from build123d import *

# Parameters (mm, degrees)
F1_DEPTH = 2.54


with BuildPart() as f1:
    # F0 (on Front) → F1 (new body, symmetric)
    with BuildSketch(Plane.XZ):
        with BuildLine():
            ThreePointArc((8.884708, -0.306712), (8.888677, -0.153379), (8.89, 0))
            ThreePointArc((8.89, 0), (8.888677, 0.153379), (8.884708, 0.306712))
            ThreePointArc((8.884708, 0.306712), (8.754941, 1.543732), (8.453796, 2.750534))
            ThreePointArc((8.453796, 2.750534), (8.353867, 3.040559), (8.243992, 3.326964))
            ThreePointArc((8.243992, 3.326964), (7.698966, 4.445), (7.003232, 5.476025))
            ThreePointArc((7.003232, 5.476025), (6.810135, 5.714382), (6.60893, 5.945935))
            ThreePointArc((6.60893, 5.945935), (5.714382, 6.810135), (4.707974, 7.541026))
            ThreePointArc((4.707974, 7.541026), (4.445, 7.698966), (4.176733, 7.847739))
            ThreePointArc((4.176733, 7.847739), (3.040559, 8.353867), (1.844866, 8.696469))
            ThreePointArc((1.844866, 8.696469), (1.543732, 8.754941), (1.240761, 8.802989))
            ThreePointArc((1.240761, 8.802989), (0, 8.89), (-1.240761, 8.802989))
            ThreePointArc((-1.240761, 8.802989), (-1.543732, 8.754941), (-1.844866, 8.696469))
            ThreePointArc((-1.844866, 8.696469), (-3.040559, 8.353867), (-4.176733, 7.847739))
            ThreePointArc((-4.176733, 7.847739), (-4.445, 7.698966), (-4.707974, 7.541026))
            ThreePointArc((-4.707974, 7.541026), (-5.714382, 6.810135), (-6.60893, 5.945935))
            ThreePointArc((-6.60893, 5.945935), (-6.810135, 5.714382), (-7.003232, 5.476025))
            ThreePointArc((-7.003232, 5.476025), (-7.698966, 4.445), (-8.243992, 3.326964))
            ThreePointArc((-8.243992, 3.326964), (-8.353867, 3.040559), (-8.453796, 2.750534))
            ThreePointArc((-8.453796, 2.750534), (-8.754941, 1.543732), (-8.884708, 0.306712))
            ThreePointArc((-8.884708, 0.306712), (-8.89, 0), (-8.884708, -0.306712))
            ThreePointArc((-8.884708, -0.306712), (-8.754941, -1.543732), (-8.453796, -2.750534))
            ThreePointArc((-8.453796, -2.750534), (-8.353867, -3.040559), (-8.243992, -3.326964))
            ThreePointArc((-8.243992, -3.326964), (-7.698966, -4.445), (-7.003232, -5.476025))
            ThreePointArc((-7.003232, -5.476025), (-6.810135, -5.714382), (-6.60893, -5.945935))
            ThreePointArc((-6.60893, -5.945935), (-5.714382, -6.810135), (-4.707974, -7.541026))
            ThreePointArc((-4.707974, -7.541026), (-4.445, -7.698966), (-4.176733, -7.847739))
            ThreePointArc((-4.176733, -7.847739), (-3.040559, -8.353867), (-1.844866, -8.696469))
            ThreePointArc((-1.844866, -8.696469), (-1.543732, -8.754941), (-1.240761, -8.802989))
            ThreePointArc((-1.240761, -8.802989), (0, -8.89), (1.240761, -8.802989))
            ThreePointArc((1.240761, -8.802989), (1.543732, -8.754941), (1.844866, -8.696469))
            ThreePointArc((1.844866, -8.696469), (3.040559, -8.353867), (4.176733, -7.847739))
            ThreePointArc((4.176733, -7.847739), (4.445, -7.698966), (4.707974, -7.541026))
            ThreePointArc((4.707974, -7.541026), (5.714382, -6.810135), (6.60893, -5.945935))
            ThreePointArc((6.60893, -5.945935), (6.810135, -5.714382), (7.003232, -5.476025))
            ThreePointArc((7.003232, -5.476025), (7.698966, -4.445), (8.243992, -3.326964))
            ThreePointArc((8.243992, -3.326964), (8.353867, -3.040559), (8.453796, -2.750534))
            ThreePointArc((8.453796, -2.750534), (8.754941, -1.543732), (8.884708, -0.306712))
        make_face()
        with BuildLine():
            ThreePointArc((-2.54, 1.684845), (3.048, 0), (-2.54, -1.684845))
            Line((-2.54, -1.684845), (-2.54, 1.684845))
        make_face(mode=Mode.SUBTRACT)
        with BuildLine():
            ThreePointArc((1.844866, 8.696469), (3.040559, 8.353867), (4.176733, 7.847739))
            Line((4.176733, 7.847739), (4.239865, 10.588624))
            Line((4.239865, 10.588624), (3.558311, 10.83669))
            Line((3.558311, 10.83669), (1.844866, 8.696469))
        make_face()
        with BuildLine():
            ThreePointArc((-1.240761, 8.802989), (0, 8.89), (1.240761, 8.802989))
            Line((1.240761, 8.802989), (0.362647, 11.400172))
            Line((0.362647, 11.400172), (-0.362647, 11.400172))
            Line((-0.362647, 11.400172), (-1.240761, 8.802989))
        make_face()
        with BuildLine():
            ThreePointArc((-4.176733, 7.847739), (-3.040559, 8.353867), (-1.844866, 8.696469))
            Line((-1.844866, 8.696469), (-3.558311, 10.83669))
            Line((-3.558311, 10.83669), (-4.239865, 10.588624))
            Line((-4.239865, 10.588624), (-4.176733, 7.847739))
        make_face()
        with BuildLine():
            ThreePointArc((-6.60893, 5.945935), (-5.714382, 6.810135), (-4.707974, 7.541026))
            Line((-4.707974, 7.541026), (-7.050085, 8.966143))
            Line((-7.050085, 8.966143), (-7.605693, 8.499933))
            Line((-7.605693, 8.499933), (-6.60893, 5.945935))
        make_face()
        with BuildLine():
            ThreePointArc((-8.243992, 3.326964), (-7.698966, 4.445), (-7.003232, 5.476025))
            Line((-7.003232, 5.476025), (-9.691514, 6.014148))
            Line((-9.691514, 6.014148), (-10.054162, 5.386024))
            Line((-10.054162, 5.386024), (-8.243992, 3.326964))
        make_face()
        with BuildLine():
            ThreePointArc((-8.884708, 0.306712), (-8.754941, 1.543732), (-8.453796, 2.750534))
            Line((-8.453796, 2.750534), (-11.164004, 2.336757))
            Line((-11.164004, 2.336757), (-11.28995, 1.622481))
            Line((-11.28995, 1.622481), (-8.884708, 0.306712))
        make_face()
        with BuildLine():
            Line((-11.164004, -2.336757), (-8.453796, -2.750534))
            ThreePointArc((-8.453796, -2.750534), (-8.754941, -1.543732), (-8.884708, -0.306712))
            Line((-8.884708, -0.306712), (-11.28995, -1.622481))
            Line((-11.28995, -1.622481), (-11.164004, -2.336757))
        make_face()
        with BuildLine():
            Line((-9.691514, -6.014148), (-7.003232, -5.476025))
            ThreePointArc((-7.003232, -5.476025), (-7.698966, -4.445), (-8.243992, -3.326964))
            Line((-8.243992, -3.326964), (-10.054162, -5.386024))
            Line((-10.054162, -5.386024), (-9.691514, -6.014148))
        make_face()
        with BuildLine():
            Line((-7.050085, -8.966143), (-4.707974, -7.541026))
            ThreePointArc((-4.707974, -7.541026), (-5.714382, -6.810135), (-6.60893, -5.945935))
            Line((-6.60893, -5.945935), (-7.605693, -8.499933))
            Line((-7.605693, -8.499933), (-7.050085, -8.966143))
        make_face()
        with BuildLine():
            Line((-3.558311, -10.83669), (-1.844866, -8.696469))
            ThreePointArc((-1.844866, -8.696469), (-3.040559, -8.353867), (-4.176733, -7.847739))
            Line((-4.176733, -7.847739), (-4.239865, -10.588624))
            Line((-4.239865, -10.588624), (-3.558311, -10.83669))
        make_face()
        with BuildLine():
            Line((4.239865, -10.588624), (4.176733, -7.847739))
            ThreePointArc((4.176733, -7.847739), (3.040559, -8.353867), (1.844866, -8.696469))
            Line((1.844866, -8.696469), (3.558311, -10.83669))
            Line((3.558311, -10.83669), (4.239865, -10.588624))
        make_face()
        with BuildLine():
            Line((7.605693, -8.499933), (6.60893, -5.945935))
            ThreePointArc((6.60893, -5.945935), (5.714382, -6.810135), (4.707974, -7.541026))
            Line((4.707974, -7.541026), (7.050085, -8.966143))
            Line((7.050085, -8.966143), (7.605693, -8.499933))
        make_face()
        with BuildLine():
            Line((10.054162, -5.386024), (8.243992, -3.326964))
            ThreePointArc((8.243992, -3.326964), (7.698966, -4.445), (7.003232, -5.476025))
            Line((7.003232, -5.476025), (9.691514, -6.014148))
            Line((9.691514, -6.014148), (10.054162, -5.386024))
        make_face()
        with BuildLine():
            Line((11.28995, -1.622481), (8.884708, -0.306712))
            ThreePointArc((8.884708, -0.306712), (8.754941, -1.543732), (8.453796, -2.750534))
            Line((8.453796, -2.750534), (11.164004, -2.336757))
            Line((11.164004, -2.336757), (11.28995, -1.622481))
        make_face()
        with BuildLine():
            ThreePointArc((7.003232, 5.476025), (7.698966, 4.445), (8.243992, 3.326964))
            Line((8.243992, 3.326964), (10.054162, 5.386024))
            Line((10.054162, 5.386024), (9.691514, 6.014148))
            Line((9.691514, 6.014148), (7.003232, 5.476025))
        make_face()
        with BuildLine():
            ThreePointArc((4.707974, 7.541026), (5.714382, 6.810135), (6.60893, 5.945935))
            Line((6.60893, 5.945935), (7.605693, 8.499933))
            Line((7.605693, 8.499933), (7.050085, 8.966143))
            Line((7.050085, 8.966143), (4.707974, 7.541026))
        make_face()
        with BuildLine():
            ThreePointArc((8.453796, 2.750534), (8.754941, 1.543732), (8.884708, 0.306712))
            Line((8.884708, 0.306712), (11.28995, 1.622481))
            Line((11.28995, 1.622481), (11.164004, 2.336757))
            Line((11.164004, 2.336757), (8.453796, 2.750534))
        make_face()
        with BuildLine():
            Line((0.362647, -11.400172), (1.240761, -8.802989))
            ThreePointArc((1.240761, -8.802989), (0, -8.89), (-1.240761, -8.802989))
            Line((-1.240761, -8.802989), (-0.362647, -11.400172))
            Line((-0.362647, -11.400172), (0.362647, -11.400172))
        make_face()
    extrude(amount=F1_DEPTH, both=True)


solid = f1.part
Model file for the job. Use its own axes, mm. A direction names the side the tool comes from. Give positions to 0.01 mm unless a question says otherwise; leave off trailing zeros. Loops run counter-clockwise (first coordinate to the right, second up) from the corner with the lowest first, then second, coordinate; pieces in that order, holes last.
1) Saw through at C-C (z = -1.25). Write the cut outline in (x, y).
2) Wall check: line 1 (Z direction, x = 0, y = -0.4); line 2 (Z direction, x = 2, y = -2.2); line 3 (X direction, y = -2, z = 1.5). Give the ranges that are in metal, low to high.
3) Tool access for faces 4 (the flat face through (-2.54, 0, 0)), 5 (the flat face through (9.1, 0, 4.3)), 6 (the flat face through (-0.796, -0.036, 10.12)), 7 (the flat face through (-2.71, -0.04, -9.78)), 8 (the flat face through (-10.1, -0.04, 0.97)): list every direction of +Z, -Z, +X, -X, +Y, -Y with a clear straight run to the whole face (end or side of a thin tool).
4) Flat gauge pins, fed straight in: pin 1 Ø1 at (x, y) = (7, 0.5) entering from +Z; pin 2 Ø5.5 at (x, z) = (0, 0) entering from -Y; pin 3 Ø1 at (y, z) = (1, 0.5) entering from +X; pin 4 Ø1 at (y, z) = (2, -5.5) entering from -X. Where does each tip first touch, or does it go through?
5) Saw through at B-B (z = -9.25). Write the cut outline in (x, y).
6) Saw through at D-D (x = -9.25). Write the cut outline in (y, z), plus the area to 3 significant figures.
7) Saw through at A-A (x = 0). Write the cut outline in (y, z).
8) Pull direction Z, two halves, no side cores. Call faces 1 (the flat face through (5.86, -0.04, -8.24)), 2 (the flat face through (9.83, -0.04, 2.54)), 3 (the flat face through (-3, -2.54, 0)): +Z half, -Z half, draft (parallel to the pull), parting line (faces both ways), or undercut.
Answer block:
1. outline: (-10.61, -2.54) - (-2.54, -2.54) - (-2.54, 2.54) - (-10.61, 2.54) - close; (2.78, -2.54) - (10.61, -2.54) - (10.61, 2.54) - (2.78, 2.54) - close
2. line 1: z = -11.4 to -3.05, 3.05 to 11.4
2. line 2: z = -8.89 to -2.3, 2.3 to 8.89
2. line 3: x = -11.07 to -2.54, 2.65 to 11.07
3. face 4: +Y, -Y
3. face 5: +X, +Y, -Y
3. face 6: +Z, +Y, -Y
3. face 7: -Z, +Y, -Y
3. face 8: -X, +Y, -Y
4. pin 1: stops at z = 8.97
4. pin 2: stops at y = -2.54
4. pin 3: stops at x = 10.15
4. pin 4: stops at x = -10.05
5. outline: (-4.21, -2.54) - (-2.29, -2.54) - (-2.29, 2.54) - (-4.21, 2.54) - close; (-1.09, -2.54) - (1.09, -2.54) - (1.09, 2.54) - (-1.09, 2.54) - close; (2.29, -2.54) - (4.21, -2.54) - (4.21, 2.54) - (2.29, 2.54) - close
6. outline: (-2.54, -5.93) - (2.54, -5.93) - (2.54, -4.47) - (-2.54, -4.47) - close; (-2.54, -2.63) - (2.54, -2.63) - (2.54, -0.51) - (-2.54, -0.51) - close; (-2.54, 0.51) - (2.54, 0.51) - (2.54, 2.63) - (-2.54, 2.63) - close; (-2.54, 4.47) - (2.54, 4.47) - (2.54, 5.93) - (-2.54, 5.93) - close
6. area: 36.3 mm2
7. outline: (-2.54, -11.4) - (2.54, -11.4) - (2.54, -3.05) - (-2.54, -3.05) - close; (-2.54, 3.05) - (2.54, 3.05) - (2.54, 11.4) - (-2.54, 11.4) - close
8. face 1: -Z half
8. face 2: undercut
8. face 3: draft
